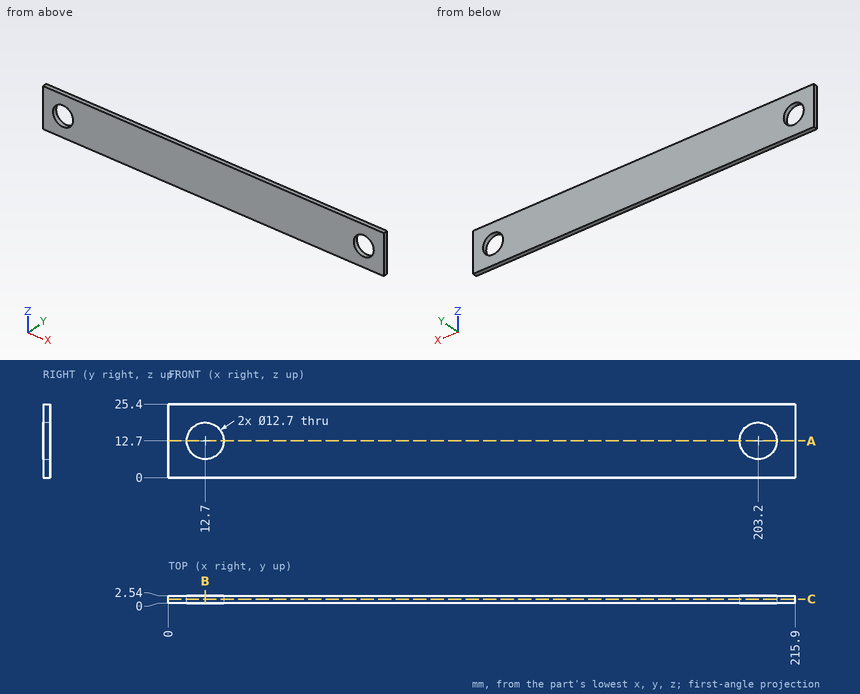
Verification items for this drawing (mm, ordinates from the low corner). Coordinates: 2 decimals unless noted, no trailing zeros. Order: outer loops, then holes, each group sorted by start corner. A loop starts at its lowest first (then second) coordinate and runs counter-clockwise, first axis right, second up. Notation, with made-up numbers: (52, 74) -> (85, 74) arc R6 ccw to (85, 79) -> close; hole circle Ø5 at (-0.75, 22.25). An arc over 180 degrees is marked (long way). Put each result on its own line as item: value. Start each with the question number.
1. Go/stop test with a flat-tipped pin: pin 1 Ø7.5 at (x, z) = (12.7, 12.7) entering from +Y. Record where the tip stops, or that it passes through.
2. Cross-section at C-C, the plane y = 1.4. Record the boundary of the cut face in (x, z).
3. Cross-section at B-B, the plane x = 12.7. Record the boundary of the cut face in (y, z), then the cut area to 3 significant figures.
4. Material ranges on L1, parallel to X at y = 0.9, z = 12.7; L2, parallel to Z at x = 203.2, y = 0.5; L3, parallel to X at y = 1.3, z = 14.5, recorded low to high. Write a range as [from, to].
5. Cross-section at A-A, the plane z = 12.7. Record the boundary of the cut face in (x, y).
Computed:
1. pin 1: through
2. outline: (0, 0) -> (215.9, 0) -> (215.9, 25.4) -> (0, 25.4) -> close; hole circle Ø12.7 at (12.7, 12.7); hole circle Ø12.7 at (203.2, 12.7)
3. outline: (0, 0) -> (2.54, 0) -> (2.54, 6.35) -> (0, 6.35) -> close; (0, 19.05) -> (2.54, 19.05) -> (2.54, 25.4) -> (0, 25.4) -> close
3. area: 32.3 mm2
4. L1: [0, 6.35], [19.05, 196.85], [209.55, 215.9]
4. L2: [0, 6.35], [19.05, 25.4]
4. L3: [0, 6.61], [18.79, 197.11], [209.29, 215.9]
5. outline: (0, 0) -> (6.35, 0) -> (6.35, 2.54) -> (0, 2.54) -> close; (19.05, 0) -> (196.85, 0) -> (196.85, 2.54) -> (19.05, 2.54) -> close; (209.55, 0) -> (215.9, 0) -> (215.9, 2.54) -> (209.55, 2.54) -> close
